The model under review builds one solid part; all positions refer to its coordinate system, in mm. Face numbers are marked on the shaded views. A direction names the side the tool comes from. Coordinates: 2 decimals unless noted, no trailing zeros. Order: outer loops, then holes, each group sorted by start corner. A loop starts at its lowest first (then second) coordinate and runs counter-clockwise, first axis right, second up. Notation, with made-up numbers: (-10.5, 55.25) -> (13.5, 55.25) arc R22 ccw to (13.5, 93.25) -> close; hole circle Ø5 at (-25.75, 69.25). An arc over 180 degrees is marked (long way). Use CSV: the item, a comma, the result in double quotes. Start each with the question number.
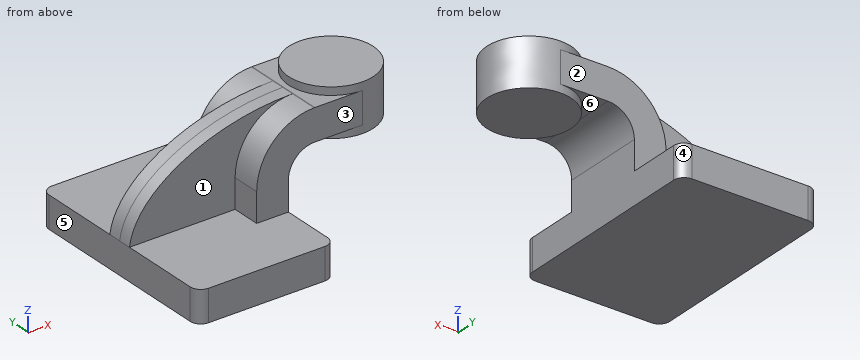
```python
from build123d import *

# Parameters (mm, degrees)
F1_DEPTH = 63.5
F2_DEPTH = 25.4
F3_DEPTH = 7.9375
F5_R     = 6.35


with BuildPart() as f1:
    # F0 (on Front) → F1 (new body, symmetric)
    with BuildSketch(Plane.XZ):
        Polygon((22.225, 9.525), (-41.275, 9.525), (-41.275, -9.525), (41.275, -9.525), (41.275, 9.525), align=None)
    extrude(amount=F1_DEPTH, both=True)

    # F0 (on Front) → F2 (join, symmetric)
    with BuildSketch(Plane.XZ):
        with BuildLine():
            Line((22.225, 27.0002), (22.225, 9.525))
            Line((22.225, 9.525), (41.275, 9.525))
            Line((41.275, 9.525), (41.275, 27.0002))
            ThreePointArc((41.275, 27.0002), (45.9246798487, 38.2255201513), (57.15, 42.8752))
            Line((57.15, 42.8752), (60.325, 42.8752))
            Line((60.325, 42.8752), (60.325, 61.9252))
            Line((60.325, 61.9252), (57.15, 61.9252))
            add(Edge.make_bspline(
                [(56.7554491642, 61.9229712909), (56.8869413618, 61.9238786407), (57.0184585552, 61.9246216516), (57.15, 61.9252)],
                knots=[111.2049462729, 111.2049462729, 111.2049462729, 111.2049462729, 111.5045361635, 111.5045361635, 111.5045361635, 111.5045361635], degree=3))
            ThreePointArc((56.7554491642, 61.9229712909), (32.3151926428, 51.5560133347), (22.225, 27.0002))
        make_face()
        Polygon((85.7297200717, 61.9252), (60.325, 61.9252), (60.325, 42.8752), (85.7486508407, 42.8752), align=None)
    extrude(amount=F2_DEPTH, both=True)

    # F0 (on Front) → F3 (join, symmetric)
    with BuildSketch(Plane.XZ):
        with BuildLine():
            add(Edge.make_bspline(
                [(-41.275, 9.525), (-37.4179048528, 38.6063461027), (7.9467836295, 61.5861715867), (56.7554491642, 61.9229712909)],
                knots=[0, 0, 0, 0, 111.2049462729, 111.2049462729, 111.2049462729, 111.2049462729], degree=3))
            Line((-41.275, 9.525), (22.225, 9.525))
            Line((22.225, 9.525), (22.225, 27.0002))
            ThreePointArc((22.225, 27.0002), (32.3151926428, 51.5560133347), (56.7554491642, 61.9229712909))
        make_face()
    extrude(amount=F3_DEPTH, both=True)

    # F0 (on Front) → F4 (revolve)
    with BuildSketch(Plane.XZ):
        Polygon((85.725, 66.675), (85.7297200717, 61.9252), (85.7486508407, 42.8752), (85.7533961535, 38.1), (111.125, 38.1), (111.125, 66.675), align=None)
    revolve(axis=Axis((85.7391980767, 0, 52.3875), (0.0009937407, 0, -0.9999995062)))

    # F5
    f5_edges = [f1.edges().sort_by_distance(p)[0] for p in [
        (41.275, 63.5, 0),
        (41.275, -63.5, 0),
        (-41.275, 63.5, 0),
        (-41.275, -63.5, 0),
    ]]
    fillet(f5_edges, radius=F5_R)


solid = f1.part
```
Q1. For the marked faces 1, 2 and 3, list the 3-axis set-ups (+Z, -Z, +X, -X, +Y, -Y) from which the entire face can be reached by the end or side of a thin tool; tool diameter is ignored.
Q2. To check wall thickness, follow probe 1 along Z at (x, y) = (67, -17.5); probe 2 along X at (y, z) = (-29, 0) (3 decimals); probe 3 along Z at (x, y) = (41, 41) (3 decimals). State the ranges of each line that lie inside material, in increasing order.
Q3. Add section A-A, the plane y = -41. State the section outline as (x, z) points (3 decimals).
Q4. Clearance check with flat-ended pins moving along their axes: pin 1 Ø10 at (y, z) = (19, 30) entering from +X; pin 2 Ø2 at (x, z) = (-21, 33) entering from +Y; pin 3 Ø11 at (y, z) = (27.5, 16.5) entering from +X (3 decimals); pin 4 Ø10 at (y, z) = (-31, 56) entering from -X. State where each tip first meets the part, or that it passes through.
Q5. Draft analysis for pull direction X (two halves, no side actions). For the marked faces 4, 5 and 6, state which applies: +X half, -X half, draft (parallel to the pull), parting line (faces both ways), or undercut.
Answer block:
1,face 1,"+Z, -X, -Y"
1,face 2,"+Z, +X, -X, +Y"
1,face 3,"+Z, +X, -X, -Y"
2,probe 1,"z = 42.88 to 61.93"
2,probe 2,"x = -41.275 to 41.275"
2,probe 3,"z = -9.525 to 9.525"
3,outline,"(-41.275, -9.525) -> (41.275, -9.525) -> (41.275, 9.525) -> (-41.275, 9.525) -> close"
4,pin 1,"stops at x = 43.44"
4,pin 2,"stops at y = 7.94"
4,pin 3,"stops at x = 41.275"
4,pin 4,"passes through"
5,face 4,"+X half"
5,face 5,"-X half"
5,face 6,"undercut"
